from build123d import *

# Parameters (mm, degrees)
BOSS_EXTRUDE1_DEPTH      = 1.9939
BOSS_EXTRUDE1_DEPTH_BACK = 1.9939
SKETCH1_R                = 5.12


with BuildPart() as part:
    # Sketch1 → Boss-Extrude1 (new, two sides: drawn at the far end of the back side and taken through both)
    with BuildSketch(Plane(origin=(0, 0, 0), x_dir=(1, 0, 0), z_dir=(0, 1, 0)).offset(-BOSS_EXTRUDE1_DEPTH_BACK)):
        Polygon((-3.592850725, 6.223), (-7.18570145, 0), (-3.592850725, -6.223), (3.592850725, -6.223), (7.18570145, 0), (3.592850725, 6.223), align=None)
        with Locations(Location((0, 0, 0), (0, 0, 270))):
            Circle(SKETCH1_R, mode=Mode.SUBTRACT)
    extrude(amount=BOSS_EXTRUDE1_DEPTH + BOSS_EXTRUDE1_DEPTH_BACK)


solid = part.part
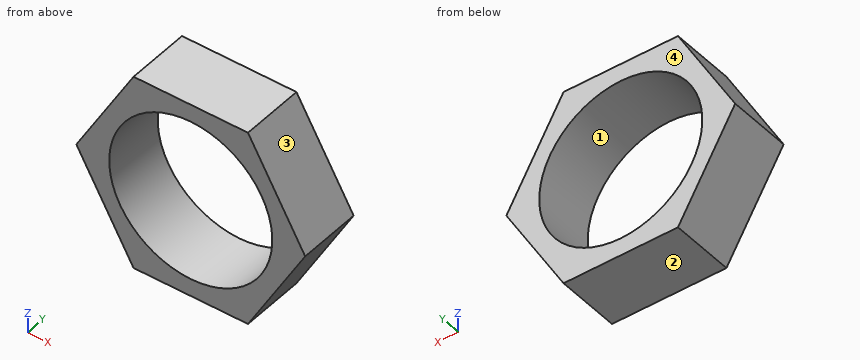
Could you check a few things on this model? Use its own coordinates, in mm. Face numbers are marked on the shaded views. Coordinates: 2 decimals unless noted, no trailing zeros. Order: outer loops, then holes, each group sorted by start corner. A loop starts at its lowest first (then second) coordinate and runs counter-clockwise, first axis right, second up.
Q1. Suppose I cut it at A-A on x = 0. Please give me the cut outline in (y, z).
Q2. Suppose I cut it at B-B on z = 4.5. Please give me the cut outline in (x, y).
Q3. Will these pins go through, and if not, where does the flat tip stop? pin 1 (1.5 mm diameter, centred on y = 1, z = 3.5, fed in from +X); pin 2 (1 mm diameter, centred on y = -1.5, z = -2.5, fed in from -X); pin 3 (2 mm diameter, centred on y = 1, z = -4.5, fed in from -X) (3 decimals).
Q4. Suppose I cut it at D-D on x = -6.25. Please give me the cut outline in (y, z).
Q5. Thinking about a two-plate mould opening in Z: for the marked faces 1, 2, 3 and 4, which applies, released by +Z, released by -Z, zero draft, split by the parting line, or undercut?
Q6. Suppose I cut it at C-C on y = 0.4. Please give me the cut outline in (x, z).
Q7. Please list where these lines run through material, in increasing order: L1, parallel to Z at x = 3.75, y = 0.85; L2, parallel to Z at x = -4, y = 1; L3, parallel to X at y = 0, z = 4.5.
Answer:
1. outline: (-1.99, -6.22) - (1.99, -6.22) - (1.99, -5.12) - (-1.99, -5.12) - close; (-1.99, 5.12) - (1.99, 5.12) - (1.99, 6.22) - (-1.99, 6.22) - close
2. outline: (-4.59, -1.99) - (-2.44, -1.99) - (-2.44, 1.99) - (-4.59, 1.99) - close; (2.44, -1.99) - (4.59, -1.99) - (4.59, 1.99) - (2.44, 1.99) - close
3. pin 1: stops at x = 5.6
3. pin 2: stops at x = -6.03
3. pin 3: stops at x = -5.165
4. outline: (-1.99, -1.62) - (1.99, -1.62) - (1.99, 1.62) - (-1.99, 1.62) - close
5. face 1: undercut
5. face 2: released by -Z
5. face 3: released by +Z
5. face 4: zero draft
6. outline: (-7.19, 0) - (-3.59, -6.22) - (3.59, -6.22) - (7.19, 0) - (3.59, 6.22) - (-3.59, 6.22) - close; hole circle Ø10.24 at (0, 0)
7. L1: z = -5.95 to -3.49, 3.49 to 5.95
7. L2: z = -5.52 to -3.2, 3.2 to 5.52
7. L3: x = -4.59 to -2.44, 2.44 to 4.59
